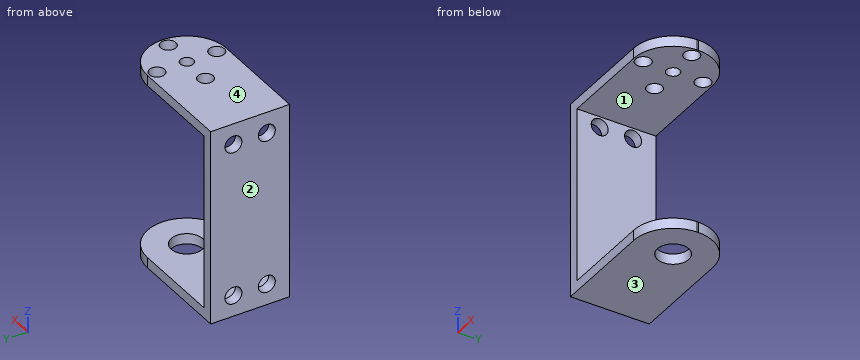
from build123d import *

# Parameters (mm, degrees)
BOSS_EXTRUDE1_DEPTH = 24.003
CUT_EXTRUDE1_DEPTH  = 68.813026147
CUT_EXTRUDE2_REACH  = 69.813
SKETCH3_R           = 2
SKETCH3_R_2         = 2.34315
CUT_EXTRUDE3_REACH  = 69.813
SKETCH4_R           = 4.7625
CUT_EXTRUDE4_REACH  = 59.49
SKETCH5_R           = 2.5868


with BuildPart() as part:
    # Sketch1 → Boss-Extrude1 (new body)
    with BuildSketch(Plane(origin=(0, 0, 0), x_dir=(1, 0, 0), z_dir=(0, 1, 0))):
        Polygon((-21.4375, -29.845), (21.4375, -29.845), (21.4375, -26.67), (-18.2625, -26.67), (-18.2625, 26.67), (21.4375, 26.67), (21.4375, 29.845), (-21.4375, 29.845), align=None)
    extrude(amount=BOSS_EXTRUDE1_DEPTH)

    # Sketch2 → Cut-Extrude1 (cut, through all)
    with BuildSketch(Plane.XY.offset(29.845)):
        with BuildLine():
            Line((112.499618931, 24.003), (15.0875, 24.003))
            Line((15.0875, 24.003), (9.4375, 24.003))
            ThreePointArc((9.4375, 24.003), (21.439, 12.0015), (9.4375, 0))
            Line((9.4375, 0), (15.0875, 0))
            Line((15.0875, 0), (112.499618931, 0))
            Line((112.499618931, 0), (307.323856793, 0))
            Line((307.323856793, 0), (307.323856793, 24.003))
            Line((307.323856793, 24.003), (112.499618931, 24.003))
        make_face()
    extrude(amount=-CUT_EXTRUDE1_DEPTH, mode=Mode.SUBTRACT)

    # Sketch3 → Cut-Extrude2 (cut, up to next)
    with BuildSketch(Plane.XY.offset(29.845), mode=Mode.PRIVATE) as cut_extrude2_sk1:
        with Locations((9.4375, 12.0015)):
            Circle(SKETCH3_R)
    cut_extrude2_tool1 = extrude(cut_extrude2_sk1.sketch, amount=-CUT_EXTRUDE2_REACH, mode=Mode.PRIVATE) & part.part
    # Sketch3 → Cut-Extrude2 (cut, up to next)
    with BuildSketch(Plane.XY.offset(29.845), mode=Mode.PRIVATE) as cut_extrude2_sk2:
        with Locations((9.4375, 21.0947)):
            Circle(SKETCH3_R_2)
    cut_extrude2_tool2 = extrude(cut_extrude2_sk2.sketch, amount=-CUT_EXTRUDE2_REACH, mode=Mode.PRIVATE) & part.part
    # Sketch3 → Cut-Extrude2 (cut, up to next)
    with BuildSketch(Plane.XY.offset(29.845), mode=Mode.PRIVATE) as cut_extrude2_sk3:
        with Locations((18.5307, 12.0015)):
            Circle(SKETCH3_R_2)
    cut_extrude2_tool3 = extrude(cut_extrude2_sk3.sketch, amount=-CUT_EXTRUDE2_REACH, mode=Mode.PRIVATE) & part.part
    # Sketch3 → Cut-Extrude2 (cut, up to next)
    with BuildSketch(Plane.XY.offset(29.845), mode=Mode.PRIVATE) as cut_extrude2_sk4:
        with Locations((9.4375, 2.9083)):
            Circle(SKETCH3_R_2)
    cut_extrude2_tool4 = extrude(cut_extrude2_sk4.sketch, amount=-CUT_EXTRUDE2_REACH, mode=Mode.PRIVATE) & part.part
    # Sketch3 → Cut-Extrude2 (cut, up to next)
    with BuildSketch(Plane.XY.offset(29.845), mode=Mode.PRIVATE) as cut_extrude2_sk5:
        with Locations((0.3443, 12.0015)):
            Circle(SKETCH3_R_2)
    cut_extrude2_tool5 = extrude(cut_extrude2_sk5.sketch, amount=-CUT_EXTRUDE2_REACH, mode=Mode.PRIVATE) & part.part
    add(cut_extrude2_tool1.solids().sort_by_distance((9.4375, 12.0015, 29.845))[0], mode=Mode.SUBTRACT)
    add(cut_extrude2_tool2.solids().sort_by_distance((9.4375, 21.0947, 29.845))[0], mode=Mode.SUBTRACT)
    add(cut_extrude2_tool3.solids().sort_by_distance((18.5307, 12.0015, 29.845))[0], mode=Mode.SUBTRACT)
    add(cut_extrude2_tool4.solids().sort_by_distance((9.4375, 2.9083, 29.845))[0], mode=Mode.SUBTRACT)
    add(cut_extrude2_tool5.solids().sort_by_distance((0.3443, 12.0015, 29.845))[0], mode=Mode.SUBTRACT)

    # Sketch4 → Cut-Extrude3 (cut, up to next)
    with BuildSketch(Plane(origin=(0, 0, -29.845), x_dir=(-1, 0, 0), z_dir=(0, 0, -1)), mode=Mode.PRIVATE) as cut_extrude3_sk1:
        with Locations((-9.4375, 12.0015)):
            Circle(SKETCH4_R)
    cut_extrude3_tool1 = extrude(cut_extrude3_sk1.sketch, amount=-CUT_EXTRUDE3_REACH, mode=Mode.PRIVATE) & part.part
    add(cut_extrude3_tool1.solids().sort_by_distance((9.4375, 12.0015, -29.845))[0], mode=Mode.SUBTRACT)

    # Sketch5 → Cut-Extrude4 (cut, up to next)
    with BuildSketch(Plane.ZY.offset(21.4375), mode=Mode.PRIVATE) as cut_extrude4_sk1:
        with Locations((-23.443, 17.0815)):
            Circle(SKETCH5_R)
    cut_extrude4_tool1 = extrude(cut_extrude4_sk1.sketch, amount=-CUT_EXTRUDE4_REACH, mode=Mode.PRIVATE) & part.part
    # Sketch5 → Cut-Extrude4 (cut, up to next)
    with BuildSketch(Plane.ZY.offset(21.4375), mode=Mode.PRIVATE) as cut_extrude4_sk2:
        with Locations((-23.443, 6.9215)):
            Circle(SKETCH5_R)
    cut_extrude4_tool2 = extrude(cut_extrude4_sk2.sketch, amount=-CUT_EXTRUDE4_REACH, mode=Mode.PRIVATE) & part.part
    # Sketch5 → Cut-Extrude4 (cut, up to next)
    with BuildSketch(Plane.ZY.offset(21.4375), mode=Mode.PRIVATE) as cut_extrude4_sk3:
        with Locations((23.443, 6.9215)):
            Circle(SKETCH5_R)
    cut_extrude4_tool3 = extrude(cut_extrude4_sk3.sketch, amount=-CUT_EXTRUDE4_REACH, mode=Mode.PRIVATE) & part.part
    # Sketch5 → Cut-Extrude4 (cut, up to next)
    with BuildSketch(Plane.ZY.offset(21.4375), mode=Mode.PRIVATE) as cut_extrude4_sk4:
        with Locations((23.443, 17.0815)):
            Circle(SKETCH5_R)
    cut_extrude4_tool4 = extrude(cut_extrude4_sk4.sketch, amount=-CUT_EXTRUDE4_REACH, mode=Mode.PRIVATE) & part.part
    add(cut_extrude4_tool1.solids().sort_by_distance((-21.4375, 17.0815, -23.443))[0], mode=Mode.SUBTRACT)
    add(cut_extrude4_tool2.solids().sort_by_distance((-21.4375, 6.9215, -23.443))[0], mode=Mode.SUBTRACT)
    add(cut_extrude4_tool3.solids().sort_by_distance((-21.4375, 6.9215, 23.443))[0], mode=Mode.SUBTRACT)
    add(cut_extrude4_tool4.solids().sort_by_distance((-21.4375, 17.0815, 23.443))[0], mode=Mode.SUBTRACT)


solid = part.part
Can you work these out from the model? Positions are in its coordinate system, mm. Face numbers are marked on the shaded views. Coordinates: 2 decimals unless noted, no trailing zeros. Loops run counter-clockwise (first coordinate to the right, second up) from the corner with the lowest first, then second, coordinate; pieces in that order, holes last. Notation, with made-up numbers: (-29, 80.5) - (-18, 80.5) arc R20 ccw to (-18, 108.5) - close; hole circle Ø2 at (88, -10.5). An arc over 180 degrees is marked (long way). Answer as a JSON object with one key per item and string values. Group by question number.
Item 1: If I drill on L1, parallel to Z at x = 18, y = 5.25 (3 decimals); L2, parallel to X at y = 10, z = -10; L3, parallel to Z at x = 8.5, y = 5 (3 decimals), over which ranges is the centre line in solid material (lowest first)? Write a range as from..to.
Item 2: If we section it at D-D (y = 8.75): List the corners of the cut face in (x, z) for me (1 decimal), plus the area to 3 significant figures.
Item 3: If we section it at A-A (x = -11): List the corners of the cut face in (y, z) for me (3 decimals), plus the area to 3 significant figures.
Item 4: For pin 1 (8.5 mm diameter, centred on y = 6.92, z = 23.44, fed in from +X); pin 2 (12 mm diameter, centred on y = 18, z = -7, fed in from +X); pin 3 (4.5 mm diameter, centred on y = 17.08, z = -23.44, fed in from +X), each with a flat end and sliding along its axis, tell me the tip position at first contact or that it passes through.
Item 5: If we section it at B-B (x = 2): List the corners of the cut face in (y, z) for me (3 decimals), plus the area to 3 significant figures.
Item 6: If we section it at C-C (z = -24.5): List the corners of the cut face in (x, y) for me, plus the area to 3 significant figures.
Item 7: If we mould it in two halves opening along Z, with no side actions, what happens to the marked faces 1, 2, 3 and 4? For each: released by +Z, released by -Z, zero draft, split by the parting line, or undercut.
Returned:
{
 "1": {"L1": "z = -29.845..-26.67, 26.67..29.845", "L2": "x = -21.44..-18.26", "L3": "z = -29.845..-26.67"},
 "2": {"outline": "(-21.4, -29.8) - (6, -29.8) - (6, -26.7) - (-18.3, -26.7) - (-18.3, -25.3) - (-21.4, -25.3) - close; (-21.4, -21.6) - (-18.3, -21.6) - (-18.3, 21.6) - (-21.4, 21.6) - close; (-21.4, 25.3) - (-18.3, 25.3) - (-18.3, 26.7) - (21, 26.7) - (21, 29.8) - (-21.4, 29.8) - close; (12.9, -29.8) - (21, -29.8) - (21, -26.7) - (12.9, -26.7) - close", "area": "393 mm²"},
 "3": {"outline": "(0, -29.845) - (24.003, -29.845) - (24.003, -26.67) - (0, -26.67) - close; (0, 26.67) - (24.003, 26.67) - (24.003, 29.845) - (0, 29.845) - close", "area": "152 mm²"},
 "4": {"pin 1": "stops at x = 21.21", "pin 2": "stops at x = -18.26", "pin 3": "passes through"},
 "5": {"outline": "(0, -29.845) - (24.003, -29.845) - (24.003, -26.67) - (0, -26.67) - close; (0, 26.67) - (10.343, 26.67) - (10.343, 29.845) - (0, 29.845) - close; (13.66, 26.67) - (24.003, 26.67) - (24.003, 29.845) - (13.66, 29.845) - close", "area": "142 mm²"},
 "6": {"outline": "(-21.44, 0) - (-18.26, 0) - (-18.26, 4.56) - (-21.44, 4.56) - close; (-21.44, 9.28) - (-18.26, 9.28) - (-18.26, 14.72) - (-21.44, 14.72) - close; (-21.44, 19.44) - (-18.26, 19.44) - (-18.26, 24) - (-21.44, 24) - close", "area": "46.2 mm²"},
 "7": {"face 1": "undercut", "face 2": "zero draft", "face 3": "released by -Z", "face 4": "released by +Z"}
}
